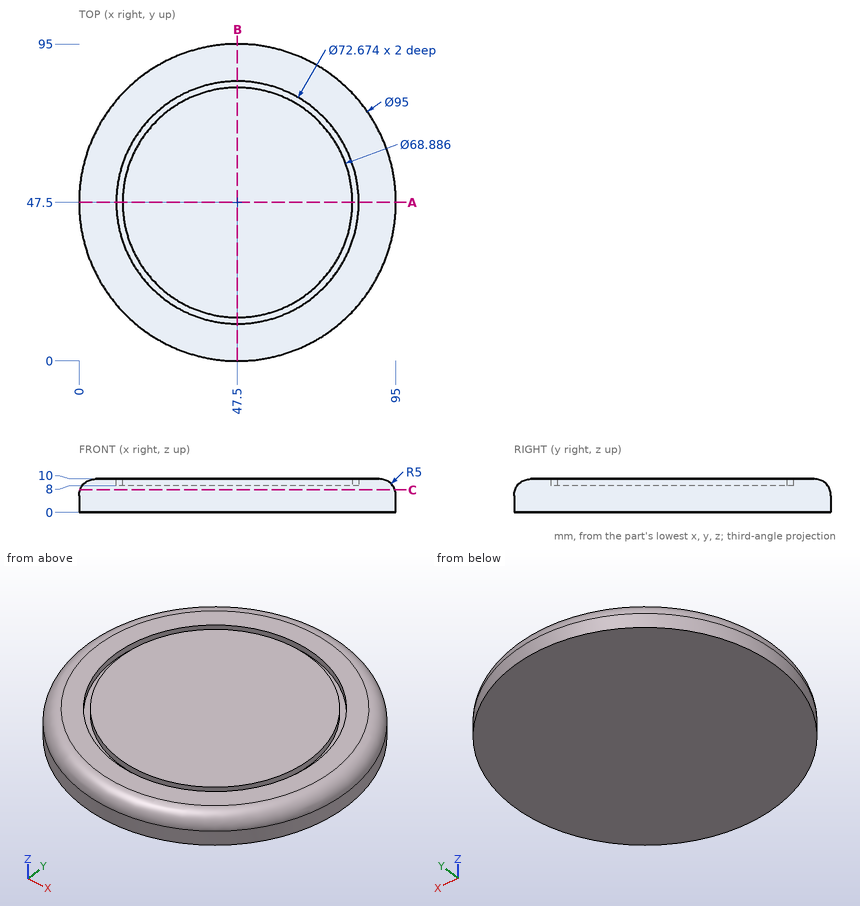
Geometry check sheet. Reference: drawing and pictorial views, mm from the part's lowest x, y, z. Coordinates: 2 decimals unless noted, no trailing zeros. Order: outer loops, then holes, each group sorted by start corner. A loop starts at its lowest first (then second) coordinate and runs counter-clockwise, first axis right, second up. Notation, with made-up numbers: (14.5, 26.5) - (46.5, 26.5) arc R12 ccw to (46.5, 32.5) - close; hole circle Ø9 at (-13, 25). An arc over 180 degrees is marked (long way). Answer in a Markdown table with one row per item. Add a question column.
1) Material ranges on line 1 along Y through (x, z) = (47.5, 9.45) (1 decimal); line 2 along Y through (x, z) = (47.5, 9.5) (1 decimal); line 3 along Y through (x, z) = (48.5, 4.25), recorded low to high. Write a range as [from, to].
2) Cross-section at A-A, the plane y = 47.5. Record the cut outline in (x, z), then the cut area to 3 significant figures.
3) Gauge pin test, flat ends, axial feed: P1, Ø1, axis at y = 71.5, z = 6.5, coming from the +X side; P2, Ø6, axis at x = 31.5, z = 2.5, coming from the +Y side; P3, Ø6, axis at y = 74.5, z = 7.5, coming from the -X side (1 decimal). Record the tip position at first contact, or that the pin passes through.
4) Cross-section at C-C, the plane z = 6.75. Record the cut outline in (x, y), then the cut area to 3 significant figures.
Check result:
| question | item | result |
|---|---|---|
| 1 | line 1 | y = [2.7, 11.2], [13.1, 81.9], [83.8, 92.3] |
| 1 | line 2 | y = [2.8, 11.2], [13.1, 81.9], [83.8, 92.2] |
| 1 | line 3 | y = [0.01, 94.99] |
| 2 | outline | (0, 0) - (95, 0) - (95, 5) arc R5 ccw to (90, 10) - (83.84, 10) - (83.84, 8) - (81.94, 8) - (81.94, 10) - (13.06, 10) - (13.06, 8) - (11.16, 8) - (11.16, 10) - (5, 10) arc R5 ccw to (0, 5) - close |
| 2 | area | 932 mm² |
| 3 | P1 | stops at x = 88.56 |
| 3 | P2 | stops at y = 93.19 |
| 3 | P3 | stops at x = 6.9 |
| 4 | outline | circle Ø94.37 at (47.5, 47.5) |
| 4 | area | 6,990 mm² |
